Drawing for the job (mm, zero at the part's lowest x, y, z). Round coordinates to 2 decimals unless told otherwise and drop trailing zeros. Loops run counter-clockwise (first coordinate to the right, second up) from the corner with the lowest first, then second, coordinate; pieces in that order, holes last. Notation, with made-up numbers: (-13.5, -38.75) - (27.5, -38.75) arc R12 cw to (27.5, -16.75) - close; hole circle Ø1 at (4.5, -8). An arc over 180 degrees is marked (long way). Put each result on its own line as item: value.
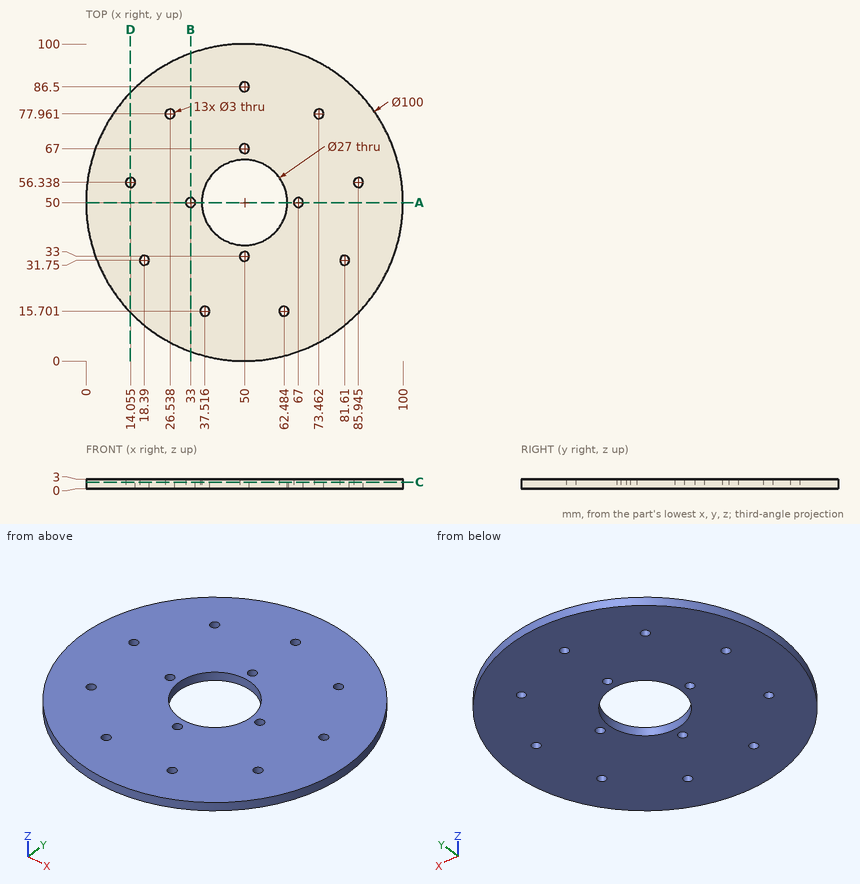
1. Band-saw the part on D-D (x = 14). List the corners of the cut face in (y, z).
A:
outline: (15.3, 0) - (54.84, 0) - (54.84, 3) - (15.3, 3) - close; (57.84, 0) - (84.7, 0) - (84.7, 3) - (57.84, 3) - close
2. Probe line 1 along Y through (x, z) = (50, 2.3); line 2 along X through (y, z) = (16.5, 1.95) (1 decimal); line 3 along X through (y, z) = (79, 0.2) (1 decimal). List the from-to ranges inside material, lowest first. Write a range as [from, to].
A:
line 1: y = [0, 31.5], [34.5, 36.5], [63.5, 65.5], [68.5, 85], [88, 100]
line 2: x = [12.9, 36.2], [38.8, 61.2], [63.8, 87.1]
line 3: x = [9.3, 25.5], [27.6, 72.4], [74.5, 90.7]
3. Pin check, flat tips, straight feed: P1, Ø3.5, axis at x = 50, y = 33, coming from the -Z side; P2, Ø2.5, axis at x = 14.05, y = 56.34, coming from the -Z side. Stop position of each tip, or through.
A:
P1: stops at z = 0
P2: passes through
4. Band-saw the part on A-A (y = 50). List the corners of the cut face in (x, z), plus the area to 3 significant figures.
A:
outline: (0, 0) - (31.5, 0) - (31.5, 3) - (0, 3) - close; (34.5, 0) - (36.5, 0) - (36.5, 3) - (34.5, 3) - close; (63.5, 0) - (65.5, 0) - (65.5, 3) - (63.5, 3) - close; (68.5, 0) - (100, 0) - (100, 3) - (68.5, 3) - close
area: 201 mm²
5. Band-saw the part on B-B (x = 33). List the corners of the cut face in (y, z).
A:
outline: (2.98, 0) - (48.5, 0) - (48.5, 3) - (2.98, 3) - close; (51.5, 0) - (97.02, 0) - (97.02, 3) - (51.5, 3) - close
6. Band-saw the part on C-C (z = 2). Give the number of separate pieces and of enclosed holes in the cut face, plus the area to 3 significant figures.
A:
separate pieces: 1
enclosed holes: 14
area: 7,190 mm²
